```python
from build123d import *

# Parameters (mm, degrees)
EXTRUDE_1_DEPTH          = 120
SKETCH_2_R               = 1.6
CUT_EXTRUDE_1_DEPTH      = 120
SKETCH_3_R               = 1.6
CUT_EXTRUDE_2_DEPTH      = 10
SKETCH_4_R               = 1.1
CUT_EXTRUDE_3_DEPTH      = 12
SKETCH_5_W               = 11
SKETCH_5_H               = 120
EXTRUDE_2_DEPTH          = 2
SKETCH_6_W               = 49
SKETCH_6_H               = 30
CUT_EXTRUDE_4_DEPTH      = 10
CUT_EXTRUDE_5_DEPTH      = 42
CUT_EXTRUDE_5_DEPTH_BACK = 16
SKETCH_7_W               = 3
SKETCH_7_H               = 30
CUT_EXTRUDE_6_DEPTH      = 35
CUT_EXTRUDE_6_DEPTH_BACK = 11
SKETCH_8_W               = 52
SKETCH_8_H               = 12
SKETCH_9_W               = 2
SKETCH_9_H               = 42
CUT_EXTRUDE_7_DEPTH      = 20
SKETCH_10_W              = 11
SKETCH_10_H              = 54
CUT_EXTRUDE_8_DEPTH      = 10
SKETCH_11_W              = 11
SKETCH_11_H              = 68
SKETCH_11_R              = 1.6
EXTRUDE_3_DEPTH          = 1
SKETCH_12_W              = 11
SKETCH_12_H              = 1
CUT_EXTRUDE_9_DEPTH      = 91
CUT_EXTRUDE_10_DEPTH     = 10
SKETCH_14_W              = 35
SKETCH_14_H              = 6
CUT_EXTRUDE_11_DEPTH     = 10
FILLET_1_R               = 2


with BuildPart() as part:
    # 草图1 → 凸台-拉伸1 (new body)
    with BuildSketch(Plane(origin=(0, 0, 0), x_dir=(1, 0, 0), z_dir=(0, 1, 0))):
        Polygon((0, 0), (8, 0), (8, -3), (-3, -3), (-3, 49), (0, 49), align=None)
    extrude(amount=EXTRUDE_1_DEPTH)

    # 草图2 → 切除-拉伸1 (cut)
    with BuildSketch(Plane(origin=(0, 0, 0), x_dir=(-1, 0, 0), z_dir=(0, 0, -1))):
        with Locations((-4.5, 60)):
            Circle(SKETCH_2_R)
        with Locations((-4.5, 45)):
            Circle(SKETCH_2_R)
        with Locations((-4.5, 30)):
            Circle(SKETCH_2_R)
        with Locations((-4.5, 15)):
            Circle(SKETCH_2_R)
        with Locations((-4.5, 75)):
            Circle(SKETCH_2_R)
        with Locations((-4.5, 90)):
            Circle(SKETCH_2_R)
        with Locations((-4.5, 105)):
            Circle(SKETCH_2_R)
    cut_extrude_1 = extrude(amount=-CUT_EXTRUDE_1_DEPTH, mode=Mode.SUBTRACT)

    # 草图3 → 切除-拉伸2 (cut)
    with BuildSketch(Plane(origin=(0, 0, 0), x_dir=(0, 0, -1), z_dir=(1, 0, 0))):
        with Locations((14.5, 7.384470662)):
            Circle(SKETCH_3_R)
        with Locations((14.5, 22.384470662)):
            Circle(SKETCH_3_R)
        with Locations((14.5, 37.384470662)):
            Circle(SKETCH_3_R)
        with Locations((14.5, 52.384470662)):
            Circle(SKETCH_3_R)
        with Locations((14.5, 67.384470662)):
            Circle(SKETCH_3_R)
        with Locations((34.5, 67.384470662)):
            Circle(SKETCH_3_R)
        with Locations((34.5, 52.384470662)):
            Circle(SKETCH_3_R)
        with Locations((34.5, 37.384470662)):
            Circle(SKETCH_3_R)
        with Locations((34.5, 22.384470662)):
            Circle(SKETCH_3_R)
        with Locations((34.5, 7.384470662)):
            Circle(SKETCH_3_R)
    extrude(amount=-CUT_EXTRUDE_2_DEPTH, mode=Mode.SUBTRACT)

    # 草图4 → 切除-拉伸3 (cut)
    with BuildSketch(Plane(origin=(0, 0, 0), x_dir=(0, 0, -1), z_dir=(1, 0, 0))):
        with Locations((15.7, 117)):
            Circle(SKETCH_4_R)
        with Locations((33.3, 117)):
            Circle(SKETCH_4_R)
        with Locations((24.5, 79.8)):
            Circle(SKETCH_4_R)
    extrude(amount=-CUT_EXTRUDE_3_DEPTH, mode=Mode.SUBTRACT)

    # 草图5 → 凸台-拉伸2 (add)
    with BuildSketch(Plane(origin=(0, 0, -49), x_dir=(-1, 0, 0), z_dir=(0, 0, -1))):
        with Locations((-2.5, 60)):
            Rectangle(SKETCH_5_W, SKETCH_5_H)
    extrude(amount=EXTRUDE_2_DEPTH)

    # 镜向3: 切除-拉伸1 across plane
    add(cut_extrude_1.mirror(Plane(origin=(0, 0, -24.5), x_dir=(1, 0, 0), z_dir=(0, 0, -1))), mode=Mode.SUBTRACT)

    # 草图6 → 切除-拉伸4 (cut)
    with BuildSketch(Plane(origin=(0, 0, 0), x_dir=(0, 0, -1), z_dir=(1, 0, 0))):
        with Locations((24.5, 15)):
            Rectangle(SKETCH_6_W, SKETCH_6_H)
    extrude(amount=-CUT_EXTRUDE_4_DEPTH, mode=Mode.SUBTRACT)

    # 草图7 → 切除-拉伸5 (cut, two sides: drawn at the far end of the back side and taken through both)
    with BuildSketch(Plane(origin=(0, 0, 0), x_dir=(0, 0, -1), z_dir=(1, 0, 0)).offset(-CUT_EXTRUDE_5_DEPTH_BACK)):
        with Locations((-1.5, 15)):
            Rectangle(SKETCH_7_W, SKETCH_7_H)
    extrude(amount=CUT_EXTRUDE_5_DEPTH + CUT_EXTRUDE_5_DEPTH_BACK, mode=Mode.SUBTRACT)

    # 草图8 → 切除-拉伸6 (cut, two sides: drawn at the far end of the back side and taken through both)
    with BuildSketch(Plane(origin=(0, 0, 0), x_dir=(0, 0, -1), z_dir=(1, 0, 0)).offset(-CUT_EXTRUDE_6_DEPTH_BACK)):
        with Locations((23, 36)):
            Rectangle(SKETCH_8_W, SKETCH_8_H)
    extrude(amount=CUT_EXTRUDE_6_DEPTH + CUT_EXTRUDE_6_DEPTH_BACK, mode=Mode.SUBTRACT)

    # 草图9 → 切除-拉伸7 (cut)
    with BuildSketch(Plane.ZY.offset(3)):
        with Locations((-50, 21)):
            Rectangle(SKETCH_9_W, SKETCH_9_H)
    extrude(amount=-CUT_EXTRUDE_7_DEPTH, mode=Mode.SUBTRACT)

    # 草图10 → 切除-拉伸8 (cut)
    with BuildSketch(Plane(origin=(0, 120, 0), x_dir=(1, 0, 0), z_dir=(0, 1, 0))):
        with Locations((2.5, 24)):
            Rectangle(SKETCH_10_W, SKETCH_10_H)
    extrude(amount=-CUT_EXTRUDE_8_DEPTH, mode=Mode.SUBTRACT)

    # 草图11 → 凸台-拉伸3 (add)
    with BuildSketch(Plane(origin=(0, 0, -51), x_dir=(-1, 0, 0), z_dir=(0, 0, -1))):
        with Locations((-2.5, 76)):
            Rectangle(SKETCH_11_W, SKETCH_11_H)
        with Locations((-4.5, 105)):
            Circle(SKETCH_11_R, mode=Mode.SUBTRACT)
        with Locations((-4.5, 45)):
            Circle(SKETCH_11_R, mode=Mode.SUBTRACT)
        with Locations((-4.5, 60)):
            Circle(SKETCH_11_R, mode=Mode.SUBTRACT)
        with Locations((-4.5, 75)):
            Circle(SKETCH_11_R, mode=Mode.SUBTRACT)
        with Locations((-4.5, 90)):
            Circle(SKETCH_11_R, mode=Mode.SUBTRACT)
    extrude(amount=EXTRUDE_3_DEPTH)

    # 草图12 → 切除-拉伸9 (cut)
    with BuildSketch(Plane(origin=(0, 110, 0), x_dir=(1, 0, 0), z_dir=(0, 1, 0))):
        with Locations((2.5, -2.5)):
            Rectangle(SKETCH_12_W, SKETCH_12_H)
    extrude(amount=-CUT_EXTRUDE_9_DEPTH, mode=Mode.SUBTRACT)

    # 草图13 → 切除-拉伸10 (cut)
    with BuildSketch(Plane.ZY.offset(3)):
        Polygon((-31.5, 66.326548237), (-24.5, 75.017418774), (-17.5, 66.326548237), (-17.5, 55.384470662), (-31.5, 55.384470662), align=None)
    extrude(amount=-CUT_EXTRUDE_10_DEPTH, mode=Mode.SUBTRACT)

    # 草图14 → 切除-拉伸11 (cut)
    with BuildSketch(Plane.ZY.offset(3)):
        with Locations((-24.5, 97.5)):
            Rectangle(SKETCH_14_W, SKETCH_14_H)
        with BuildLine():
            Line((-22.018065271, 79.5), (-7, 79.5))
            Line((-7, 79.5), (-7, 85.5))
            Line((-7, 85.5), (-42, 85.5))
            Line((-42, 85.5), (-42, 79.5))
            Line((-42, 79.5), (-26.981934729, 79.5))
            ThreePointArc((-26.981934729, 79.5), (-24.5, 82.3), (-22.018065271, 79.5))
        make_face()
    extrude(amount=-CUT_EXTRUDE_11_DEPTH, mode=Mode.SUBTRACT)

    # 圆角1
    fillet_1_edges = [part.edges().sort_by_distance(p)[0] for p in [
        (-1.5, 55.384470662, -31.5),
        (-1.5, 66.326548237, -31.5),
        (-1.5, 75.017418774, -24.5),
        (-1.5, 66.326548237, -17.5),
        (-1.5, 55.384470662, -17.5),
        (-1.5, 100.5, -7),
        (-1.5, 94.5, -7),
        (-1.5, 94.5, -42),
        (-1.5, 100.5, -42),
        (-1.5, 85.5, -7),
        (-1.5, 79.5, -7),
        (-1.5, 79.5, -22.018065271),
        (-1.5, 79.5, -26.981934729),
        (-1.5, 79.5, -42),
        (-1.5, 85.5, -42),
    ]]
    fillet(fillet_1_edges, radius=FILLET_1_R)


solid = part.part
```
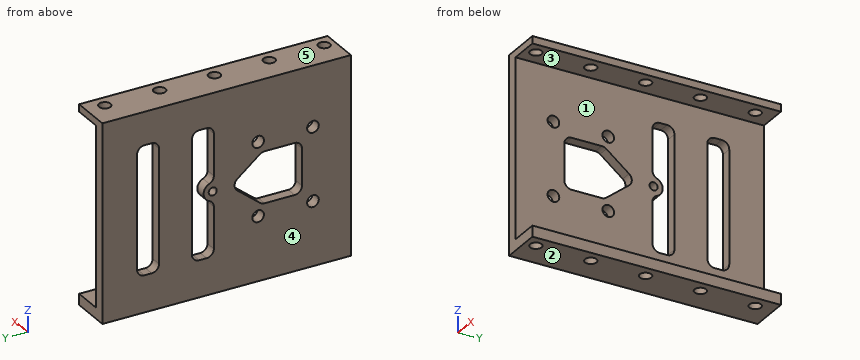
Geometry: final body of the model. Coordinates: model frame, mm. Face numbers are marked on the shaded views. A direction names the side the tool comes from. Give positions to 0.01 mm unless a question says otherwise; leave off trailing zeros. Loops run counter-clockwise (first coordinate to the right, second up) from the corner with the lowest first, then second, coordinate; pieces in that order, holes last. Notation, with made-up numbers: (75.5, 33.5) -> (115.5, 33.5) arc R22 cw to (115.5, 53.5) -> close; hole circle Ø8 at (-21, 7.5). An arc over 180 degrees is marked (long way). Use one line per item in the form item = value.
Item 1: Section query B-B on y = 60. Output: boundary loops of the cut face in (x, z).
A:
outline = (-3, -52) -> (2.9, -52) -> (2.9, -49) -> (0, -49) -> (0, -31.5) -> (-3, -31.5) -> close; (-3, -17.5) -> (0, -17.5) -> (0, 0) -> (2.9, 0) -> (2.9, 2) -> (-3, 2) -> close; (6.1, -52) -> (8, -52) -> (8, -49) -> (6.1, -49) -> close; (6.1, 0) -> (8, 0) -> (8, 2) -> (6.1, 2) -> close
Item 2: Pin query (flat end, axial travel): P1, Ø6, axis at y = 62.5, z = -30.5, coming from the +X side. Return the tip coordinate at first contact, or that it passes through.
A:
P1 = 0
Item 3: Section query D-D on z = -24.5. Output: boundary loops of the cut face in (x, y).
A:
outline = (-3, 42) -> (0, 42) -> (0, 55.38) -> (-3, 55.38) -> close; (-3, 73.83) -> (0, 73.83) -> (0, 78.7) -> (-3, 78.7) -> close; (-3, 80.9) -> (0, 80.9) -> (0, 82.3) -> (-3, 82.3) -> close; (-3, 85.5) -> (0, 85.5) -> (0, 94.5) -> (-3, 94.5) -> close; (-3, 100.5) -> (0, 100.5) -> (0, 110) -> (-3, 110) -> close
Item 4: Draft query along Z for the marked faces 3, 4 and 5. Return one class per face: pulls with the +Z half, pulls with the -Z half, needs draft (parallel to the pull), parting line crosses it, or undercut.
A:
face_3 = undercut
face_4 = needs draft
face_5 = pulls with the +Z half
Item 5: Section query C-C on y = 75. Output: boundary loops of the cut face in (x, z).
A:
outline = (-3, -52) -> (2.9, -52) -> (2.9, -49) -> (0, -49) -> (0, 0) -> (2.9, 0) -> (2.9, 2) -> (-3, 2) -> close; (6.1, -52) -> (8, -52) -> (8, -49) -> (6.1, -49) -> close; (6.1, 0) -> (8, 0) -> (8, 2) -> (6.1, 2) -> close
Item 6: Access query for the marked faces 1 and 2. Directions: +Z, -Z, +X, -X, +Y, -Y. A direction counts if a zero-diameter tool reaches every point of the face in a straight line with its end or side. Return the directions, or none.
A:
face_1 = +X, +Y, -Y
face_2 = -Z, +X, -X, +Y, -Y
Item 7: Line query: probe 1 along Y at (x, z) = (-2, -24.5); probe 2 along Y at (x, z) = (4.5, 1.3); probe 3 along Y at (x, z) = (-1.5, -37.5). Output: solid intervals per line, ascending.
A:
probe_1 = 42 to 55.38, 73.83 to 78.7, 80.9 to 82.3, 85.5 to 94.5, 100.5 to 110
probe_2 = 42 to 43.4, 46.6 to 58.4, 61.6 to 73.4, 76.6 to 88.4, 91.6 to 103.4, 106.6 to 110
probe_3 = 42 to 79.5, 85.5 to 94.5, 100.5 to 110
Item 8: Section query A-A on z = -34.5. Output: boundary loops of the cut face in (x, y), and give its area (3 significant figures).
A:
outline = (-3, 42) -> (0, 42) -> (0, 50.78) -> (-3, 50.78) -> close; (-3, 53.98) -> (0, 53.98) -> (0, 65.78) -> (-3, 65.78) -> close; (-3, 68.98) -> (0, 68.98) -> (0, 79.5) -> (-3, 79.5) -> close; (-3, 85.5) -> (0, 85.5) -> (0, 94.5) -> (-3, 94.5) -> close; (-3, 100.5) -> (0, 100.5) -> (0, 110) -> (-3, 110) -> close
area = 149 mm^2
